Verification items for the finished model (mm, model axes). Face numbers are marked on the shaded views. A direction names the side the tool comes from. Round coordinates to 2 decimals unless told otherwise and drop trailing zeros. Order: outer loops, then holes, each group sorted by start corner. A loop starts at its lowest first (then second) coordinate and runs counter-clockwise, first axis right, second up. Notation, with made-up numbers: M -20,-30.5 L 2,-30.5 A16 ccw 2,-1.5 Z; hole C -8.5,29 d9. An arc over 180 degrees is marked long. Use one line per item in the form item = value. Start each with the question number.
Item 1: Cross-section at C-C on z = 0. Enter the section's corners in (x, y), then the cut area to 3 significant figures.
Item 2: Cross-section at B-B on x = 13.5. Enter the section's corners in (y, z).
Item 3: Cross-section at A-A on y = 0. Enter the section's corners in (x, z), then the cut area to 3 significant figures.
Item 4: Cross-section at D-D on z = -33. Enter the section's corners in (x, y), then the cut area to 3 significant figures.
Item 5: Release check for a two-part mould opening along Y. For the marked faces 3, 4, 5 and 6 record: +Y half, -Y half, draft (parallel to the pull), parting line (faces both ways), or undercut.
Item 6: Go/stop test with flat-tipped pins: pin 1 Ø5 at (y, z) = (42, 5.5) entering from +X; pin 2 Ø23 at (y, z) = (15, -6) entering from +X; pin 3 Ø3.5 at (x, y) = (9.5, -45) entering from -Z. Record where each tip stops, or that it passes through.
Item 7: Tool access check on the marked faces 1 and 2. Record the directions out of +Z, -Z, +X, -X, +Y, -Y that give a thin tool (end or side, any length) a straight path to the whole face; none if there is none.
Item 8: Thickness scan on probe 1 along Z at (x, y) = (9, 42); probe 2 along Z at (x, y) = (3, 11.5); probe 3 along Y at (x, z) = (26, -28.5). Record the ranges inside material, lowest first. Write a range as [from, to].
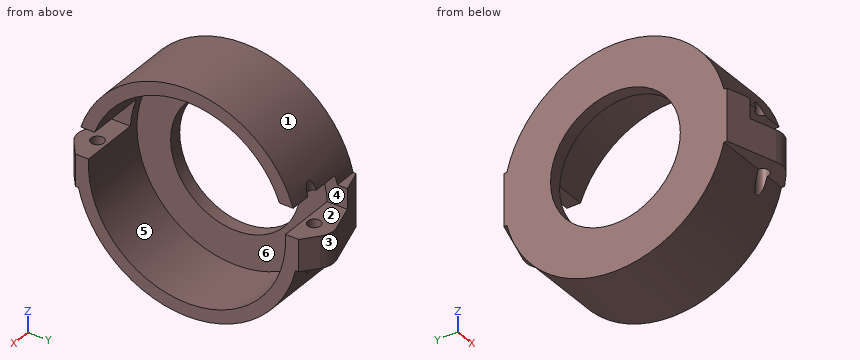
from build123d import *

# Parameters (mm, degrees)
BOSS_EXTRUDE1_DEPTH     = 10
SKETCH4_R               = 2.5
CUT_EXTRUDE1_DEPTH      = 73.697811944
CUT_EXTRUDE2_REACH      = 109.281
CUT_EXTRUDE2_END_RADIUS = 38
SKETCH5_W               = 23.074324902
SKETCH5_H               = 11


with BuildPart() as part:
    # Sketch1 → Revolve1 (revolve)
    with BuildSketch(Plane.XY, mode=Mode.PRIVATE) as revolve1_sk:
        Polygon((5, -38), (5, -25), (0, -25), (0, -43), (31.8, -43), (31.8, -38), align=None)
    revolve(revolve1_sk.sketch.rotate(Axis((96.017453448, 0, 0), (-1, 0, 0)), 180), axis=Axis((96.017453448, 0, 0), (-1, 0, 0)))

    # Sketch3 → Boss-Extrude1 (add, symmetric)
    with BuildSketch(Plane.XY):
        with BuildLine():
            Line((31.8, -43), (26.114355816, -47.581512833))
            ThreePointArc((26.114355816, -47.581512833), (22.82386933, -49.10680541), (19.202406183, -48.909768758))
            Line((19.202406183, -48.909768758), (0, -43))
            Line((0, -43), (0, -38))
            Line((0, -38), (31.8, -38))
            Line((31.8, -38), (31.8, -43))
        make_face()
    boss_extrude1 = extrude(amount=BOSS_EXTRUDE1_DEPTH, both=True)

    # Sketch4 → Cut-Extrude1 (cut, symmetric)
    with BuildSketch(Plane.XY):
        with Locations(Location((21.408505666, -41.741566399, 0), (0, 0, 358.178124169))):
            Circle(SKETCH4_R)
    cut_extrude1 = extrude(amount=CUT_EXTRUDE1_DEPTH, both=True, mode=Mode.SUBTRACT)

    # Cut-Extrude2: up to this cylinder (the profile starts outside it)
    cut_extrude2_end = Plane(origin=(20.262838, 0, 0), z_dir=(1, 0, 0)) * Cylinder(CUT_EXTRUDE2_END_RADIUS, 295.562, mode=Mode.PRIVATE)
    # Sketch5 → Cut-Extrude2 (cut, up to the surface)
    with BuildSketch(Plane(origin=(0, -50, 0), x_dir=(1, 0, 0), z_dir=(0, 1, 0)), mode=Mode.PRIVATE) as cut_extrude2_sk1:
        with Locations((20.262837549, -7.731366933)):
            Rectangle(SKETCH5_W, SKETCH5_H)
    cut_extrude2_tool1 = extrude(cut_extrude2_sk1.sketch, amount=CUT_EXTRUDE2_REACH, mode=Mode.PRIVATE) - cut_extrude2_end
    cut_extrude2 = cut_extrude2_tool1.solids().sort_by_distance((20.262838, -50, 7.731367))[0]
    add(cut_extrude2, mode=Mode.SUBTRACT)

    # Mirror1: Boss-Extrude1, Cut-Extrude1, Cut-Extrude2 across plane
    add(boss_extrude1.mirror(Plane.ZX))
    add(cut_extrude1.mirror(Plane.ZX), mode=Mode.SUBTRACT)
    add(cut_extrude2.mirror(Plane.ZX), mode=Mode.SUBTRACT)


solid = part.part
Output values:
q1.outline = M 0,-43 L 19.2,-48.91 A7.5 ccw 26.11,-47.58 L 31.8,-43 L 31.8,-38 L 5,-38 L 5,-25 L 0,-25 Z; M 0,25 L 5,25 L 5,38 L 31.8,38 L 31.8,43 L 26.11,47.58 A7.5 ccw 19.2,48.91 L 0,43 Z; hole C 21.41,-41.74 d5; hole C 21.41,41.74 d5
q1.area = 629 mm2
q2.outline = M -47.15,-10 L -41.82,-10 A43 ccw 41.82,-10 L 47.15,-10 L 47.15,2.23 L 37.93,2.23 A38 cw long -37.93,2.23 L -47.15,2.23 Z; M -40.91,13.23 L -35.62,13.23 A38 cw 35.62,13.23 L 40.91,13.23 A43 ccw Z
q3.outline = M 0,-43 L 31.8,-43 L 31.8,-38 L 5,-38 L 5,-25 L 0,-25 Z; M 0,25 L 5,25 L 5,38 L 31.8,38 L 31.8,43 L 0,43 Z
q3.area = 448 mm2
q4.outline = M 0,-27.57 L 31.8,-27.57 L 31.8,-18.84 L 5,-18.84 L 5,18.84 L 31.8,18.84 L 31.8,27.57 L 0,27.57 Z
q4.area = 743 mm2
q5.face_3 = +Y half
q5.face_4 = draft
q5.face_5 = undercut
q5.face_6 = undercut
q6.pin_1 = 8.73
q6.pin_2 = 5
q6.pin_3 = -10
q7.face_1 = +Z, +X, -X
q7.face_2 = +X, +Y, -Y
q8.probe_1 = [-10, 2.23]
q8.probe_2 = [-41.43, -22.2], [22.2, 41.43]
q8.probe_3 = [-32.2, -25.13], [25.13, 32.2]
